Verification items for the finished model (mm, model axes). Give positions to 0.01 mm unless a question says otherwise; leave off trailing zeros. Order: outer loops, then holes, each group sorted by start corner. A loop starts at its lowest first (then second) coordinate and runs counter-clockwise, first axis right, second up. Notation, with made-up numbers: (-24, -20.5) - (0, -20.5) arc R17 ccw to (0, -9.5) - close; hole circle Ø5 at (-27.75, 58.5). An arc over 180 degrees is marked (long way). Answer as a JSON object with one key per item and string values. Group by question number.
(1) Depth check by flat-ended pin: pin 1 Ø1.3 at (y, z) = (1.5, 20.5) entering from -X; pin 2 Ø2.5 at (x, z) = (21, -15) entering from -Y. Enter the tip coordinate at first touch or a pass-through.
(2) Section check C-C (y = 1.7). Record the boundary of the cut face in (x, z), then the cut area to 3 significant figures.
(3) Section check B-B (z = -15). Record the boundary of the cut face in (x, y).
(4) Section check D-D (x = 21). Record the boundary of the cut face in (y, z), then the cut area to 3 significant figures.
(5) Thickness scan on line 1 (X direction, y = 2.4, z = -15); line 2 (X direction, y = 3.9, z = -15.5); line 3 (Z direction, x = -21, y = 3.45). Record the ranges inside material, lowest first.
(6) Section check A-A (x = -16.5). Record the boundary of the cut face in (y, z), then the cut area to 4 significant figures.
```python
from build123d import *

# Parameters (mm, degrees)
SKETCH1_R           = 2.1
BOSS_EXTRUDE1_DEPTH = 4.5
CUT_EXTRUDE1_DEPTH  = 10


with BuildPart() as part:
    # Sketch1 → Boss-Extrude1 (new body)
    with BuildSketch(Plane(origin=(0, 0, 0), x_dir=(1, 0, 0), z_dir=(0, 1, 0))):
        Polygon((20, 40), (50, 25), (50, -25), (-50, -25), (-50, 25), (-20, 40), (0, 40), align=None)
        with Locations((-41, 15)):
            Circle(SKETCH1_R, mode=Mode.SUBTRACT)
        with Locations((41, 15)):
            Circle(SKETCH1_R, mode=Mode.SUBTRACT)
        with Locations((-21, 15)):
            Circle(SKETCH1_R, mode=Mode.SUBTRACT)
        with Locations((21, 15)):
            Circle(SKETCH1_R, mode=Mode.SUBTRACT)
    extrude(amount=BOSS_EXTRUDE1_DEPTH)

    # Sketch2 → Cut-Extrude1 (cut)
    with BuildSketch(Plane(origin=(0, 4.5, 0), x_dir=(1, 0, 0), z_dir=(0, 1, 0))):
        Polygon((-50, -19), (-50, -25), (-25, -25), (-25, -19), (0, -19), (0, -13), (-50, -13), align=None)
    extrude(amount=-CUT_EXTRUDE1_DEPTH, mode=Mode.SUBTRACT)


solid = part.part
```
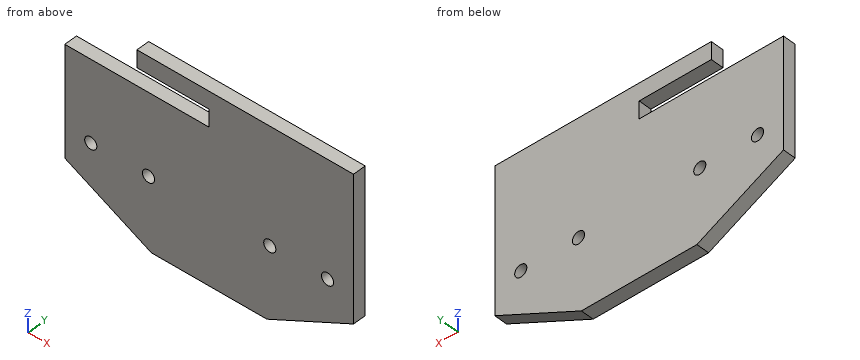
Solutions:
{
 "1": {"pin 1": "stops at x = -25", "pin 2": "passes through"},
 "2": {"outline": "(-50, -25) - (-20, -40) - (20, -40) - (50, -25) - (50, 25) - (-25, 25) - (-25, 19) - (0, 19) - (0, 13) - (-50, 13) - close; hole circle Ø4.2 at (-41, -15); hole circle Ø4.2 at (-21, -15); hole circle Ø4.2 at (21, -15); hole circle Ø4.2 at (41, -15)", "area": "5,540 mm2"},
 "3": {"outline": "(-50, 0) - (-43.1, 0) - (-43.1, 4.5) - (-50, 4.5) - close; (-38.9, 0) - (-23.1, 0) - (-23.1, 4.5) - (-38.9, 4.5) - close; (-18.9, 0) - (18.9, 0) - (18.9, 4.5) - (-18.9, 4.5) - close; (23.1, 0) - (38.9, 0) - (38.9, 4.5) - (23.1, 4.5) - close; (43.1, 0) - (50, 0) - (50, 4.5) - (43.1, 4.5) - close"},
 "4": {"outline": "(0, -39.5) - (4.5, -39.5) - (4.5, -17.1) - (0, -17.1) - close; (0, -12.9) - (4.5, -12.9) - (4.5, 25) - (0, 25) - close", "area": "271 mm2"},
 "5": {"line 1": "x = -50 to -43.1, -38.9 to -23.1, -18.9 to 18.9, 23.1 to 38.9, 43.1 to 50", "line 2": "x = -50 to -43.04, -38.96 to -23.04, -18.96 to 18.96, 23.04 to 38.96, 43.04 to 50", "line 3": "z = -39.5 to -17.1, -12.9 to 13, 19 to 25"},
 "6": {"outline": "(0, -40) - (4.5, -40) - (4.5, 13) - (0, 13) - close; (0, 19) - (4.5, 19) - (4.5, 25) - (0, 25) - close", "area": "265.5 mm2"}
}
